Build history of the part. All positions in model axes, mm. Give positions to 0.01 mm unless a question says otherwise; leave off trailing zeros. Order: outer loops, then holes, each group sorted by start corner. A loop starts at its lowest first (then second) coordinate and runs counter-clockwise, first axis right, second up. Notation, with made-up numbers: (-14, -35.5) - (28, -35.5) arc R18 cw to (28, -25.5) - close; hole circle Ø5 at (48, 67.5). An arc over 180 degrees is marked (long way). Write each question's results on one line, items separated by ' | '. Start each with the question number.
1) Drill centre lines: line 1 along Y through (x, z) = (99, 2.95); line 2 along X through (y, z) = (3406, 1.85); line 3 along Y through (x, z) = (25.5, 0.55). Where is each one in solid material? Low to high. Write a range as from..to.
2) Cut at B-B on x = 15.5. List the corners of the cut face in (y, z).
3) Drop a flat-ended pin along its axis: pin 1 Ø1.2 at (y, z) = (3407, 1.5) entering from +X. Give the stop position or say it passes through.
4) Cut at C-C on y = 3972. List the corners of the cut face in (x, z), plus the area to 3 significant figures.
5) Cut at A-A on z = 1.75. List the corners of the cut face in (x, y).
Autodesk Inventor part; units mm, degrees
ref_plane "YZ Plane" through (0, 0, 0) normal (1, 0, 0) x (0, 1, 0)
ref_plane "XZ Plane" through (0, 0, 0) normal (0, 1, 0) x (-1, 0, 0)
ref_plane "XY Plane" through (0, 0, 0) normal (0, 0, 1) x (1, 0, 0)
sketch "Sketch1" plane through (0, 0, 0) normal (0, 0, 1) x (1, 0, 0)
  line L0 (0, 0) -> (0, 4438.8737)
  line L1 (0, 4438.8737) -> (100, 4438.8737)
  line L2 (100, 4438.8737) -> (200, 0)
  line L3 (200, 0) -> (0, 0)
  circle A0 centre (0, 0) radius 30
  line L4 (0, 1479.6246) -> (166.6667, 1479.6246)
  line L5 (0, 2959.2492) -> (133.3333, 2959.2492)
  circle A1 centre (0, 1479.6246) radius 30
  circle A2 centre (0, 2959.2492) radius 30
  line L6 (190.8761, 405) -> (120.8761, 405)
  line L7 (120.8761, 405) -> (120.8761, 410)
  line L8 (120.8761, 410) -> (190.8761, 410)
  line L9 (190.8761, 410) -> (190.8761, 405)
  line L10 (109.6148, 909.8732) -> (179.6148, 909.8732)
  line L11 (179.6148, 904.8732) -> (109.6148, 904.8732)
  line L12 (109.6148, 904.8732) -> (109.6148, 909.8732)
  line L13 (179.6148, 909.8732) -> (179.6148, 904.8732)
  line L14 (98.3535, 1409.7463) -> (168.3535, 1409.7463)
  line L15 (168.3535, 1404.7463) -> (98.3535, 1404.7463)
  line L16 (98.3535, 1404.7463) -> (98.3535, 1409.7463)
  line L17 (168.3535, 1409.7463) -> (168.3535, 1404.7463)
  line L18 (87.0923, 1909.6195) -> (157.0923, 1909.6195)
  line L19 (157.0923, 1904.6195) -> (87.0923, 1904.6195)
  line L20 (87.0923, 1904.6195) -> (87.0923, 1909.6195)
  line L21 (157.0923, 1909.6195) -> (157.0923, 1904.6195)
  line L22 (75.831, 2409.4927) -> (145.831, 2409.4927)
  line L23 (145.831, 2404.4927) -> (75.831, 2404.4927)
  line L24 (75.831, 2404.4927) -> (75.831, 2409.4927)
  line L25 (145.831, 2409.4927) -> (145.831, 2404.4927)
  line L26 (64.5698, 2909.3658) -> (134.5698, 2909.3658)
  line L27 (134.5698, 2904.3658) -> (64.5698, 2904.3658)
  line L28 (64.5698, 2904.3658) -> (64.5698, 2909.3658)
  line L29 (134.5698, 2909.3658) -> (134.5698, 2904.3658)
  line L30 (53.3085, 3409.239) -> (123.3085, 3409.239)
  line L31 (123.3085, 3404.239) -> (53.3085, 3404.239)
  line L32 (53.3085, 3404.239) -> (53.3085, 3409.239)
  line L33 (123.3085, 3409.239) -> (123.3085, 3404.239)
  line L34 (42.0472, 3909.1122) -> (112.0472, 3909.1122)
  line L35 (112.0472, 3904.1122) -> (42.0472, 3904.1122)
  line L36 (42.0472, 3904.1122) -> (42.0472, 3909.1122)
  line L37 (112.0472, 3909.1122) -> (112.0472, 3904.1122)
  line L38 (0, 1629.6246) -> (163.2874, 1629.6246)
  line L39 (0, 3079.2492) -> (130.6299, 3079.2492)
  point P0 (30, 2959.2492)
  point P1 (0, 2929.2492)
  point P2 (0, 1509.6246)
  point P3 (0, 1449.6246)
  point P4 (0, 30)
  point P5 (30, 0)
  point P6 (190.7634, 410)
  point P7 (179.5022, 909.8732)
  point P8 (168.3535, 1404.7463)
  point P9 (168.2409, 1409.7463)
  point P10 (30, 1479.6246)
  point P11 (157.0923, 1904.6195)
  point P12 (156.9796, 1909.6195)
  point P13 (145.831, 2404.4927)
  point P14 (145.7184, 2409.4927)
  point P15 (134.5698, 2904.3658)
  point P16 (134.4571, 2909.3658)
  point P17 (0, 2989.2492)
  point P18 (123.3085, 3404.239)
  point P19 (123.1959, 3409.239)
  point P20 (112.0472, 3904.1122)
  point P21 (111.9346, 3909.1122)
  dimension "d65" = 100
  dimension "d67" = 200
  dimension "d68" = 60
  dimension "d69" = 1480
  dimension "d70" = 1480
  dimension "d71" = 1480
  dimension "d72" = 5
  dimension "d73" = 70
  dimension "d74" = 410
  dimension "d77" = 500
  dimension "d82" = 120
  dimension "d83" = 150
extrude "Plate3" add sketch "Sketch1" along normal blind 4 contours L39 L2 L5 A2 L0 | L0 L1 L2 L34 L36 L35 L30 L32 L31 L39
chamfer "Corner Chamfer2" distance 3 angle 45 4 edges at (123.3085, 3404.239, 2) (123.1959, 3409.239, 2) (112.0472, 3904.1122, 2) (111.9346, 3909.1122, 2)
equation "\"BendRadius\" = Thickness"
equation "\"BendReliefWidth\" = Thickness"
equation "\"BendReliefDepth\" = 0.5 * Thickness"
equation "\"CornerReliefSize\" = 4 * Thickness"
equation "\"MinimumRemnant\" = 2 * Thickness"
equation "\"TransitionRadius\" = BendRadius"
equation "\"JacobiRadiusSize\" = BendRadius"
equation "\"GapSize\" = Thickness"
properties part number "GBK 3311 central third rib_CPY" material "Steel"
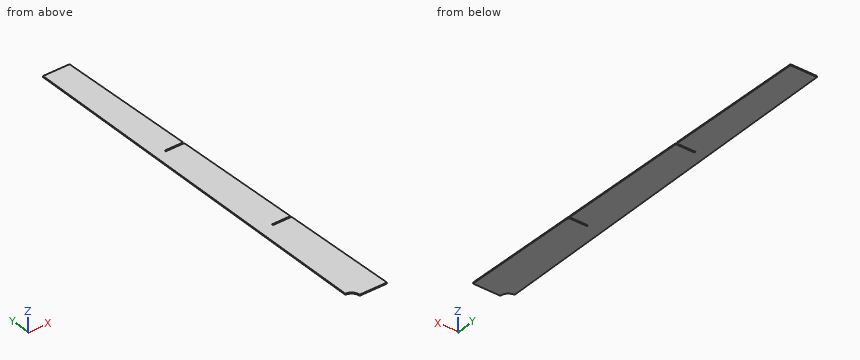
Results:
1) line 1: 2959.25..3404.24, 3409.24..3904.11, 3909.11..4438.87 | line 2: 0..53.31 | line 3: 2975.05..4438.87
2) outline: (2984.93, 0) - (4438.87, 0) - (4438.87, 4) - (2984.93, 4) - close
3) pin 1: x = 53.31
4) outline: (0, 0) - (110.52, 0) - (110.52, 4) - (0, 4) - close | area: 442 mm^2
5) outline: (0, 2989.25) arc R30 cw to (30, 2959.25) - (133.33, 2959.25) - (123.38, 3401.24) - (120.31, 3404.24) - (53.31, 3404.24) - (53.31, 3409.24) - (120.2, 3409.24) - (123.13, 3412.24) - (112.11, 3901.11) - (109.05, 3904.11) - (42.05, 3904.11) - (42.05, 3909.11) - (108.93, 3909.11) - (111.87, 3912.11) - (100, 4438.87) - (0, 4438.87) - close
